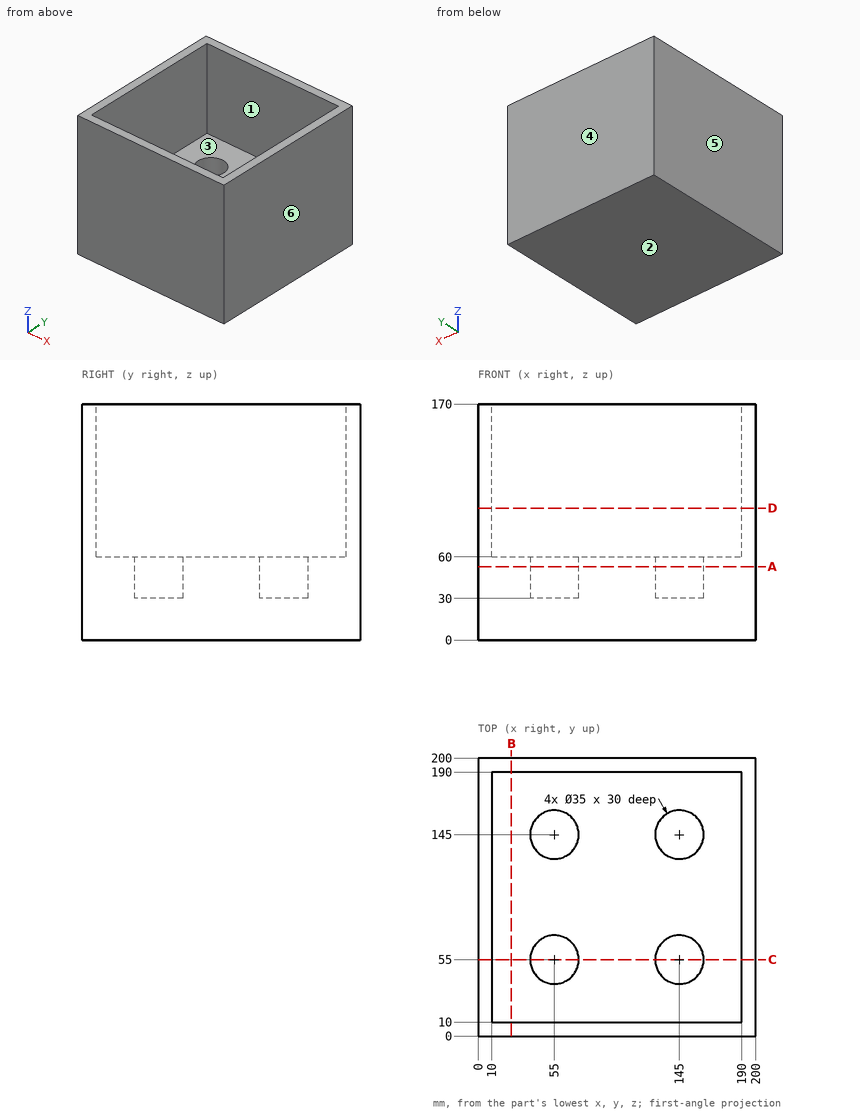
Print and shaded views of the part. All mm, measured from the part's lowest x, y and z. A direction names the side the tool comes from. Coordinates: 2 decimals unless noted, no trailing zeros. Loops run counter-clockwise (first coordinate to the right, second up) from the corner with the lowest first, then second, coordinate; pieces in that order, holes last. Notation, with made-up numbers: (67.5, -27) -> (81.5, -27) arc R33 cw to (81.5, 9) -> close; hole circle Ø6 at (23, 42). An arc over 180 degrees is marked (long way). Use a Markdown table: item, result. Add a question column.
Item 1: Band-saw the part on C-C on y = 55. Write the cut outline in (x, z), plus the area to 3 significant figures.
Item 2: Band-saw the part on B-B on x = 24. Write the cut outline in (y, z), plus the area to 3 significant figures.
Item 3: Probe probe 1 along Y at (x, z) = (145, 45); probe 2 along Y at (x, z) = (18, 112). List the from-to ranges inside material, lowest first.
Item 4: Band-saw the part on A-A on z = 53. Write the cut outline in (x, y).
Item 5: Band-saw the part on D-D on z = 95. Write the cut outline in (x, y), plus the area to 3 significant figures.
Item 6: Flat gauge pins, fed straight in: P1, Ø10.5, axis at x = 146, y = 51, coming from the +Z side; P2, Ø4, axis at x = 26, y = 57, coming from the +Z side. Where does each tip first touch, or does it go through?
Item 7: Pull direction X, two halves, no side cores. Call the marked faces 3, 4, 5 and 6: +X half, -X half, draft (parallel to the pull), parting line (faces both ways), or undercut.
Item 8: Which spindle directions (+Z, -Z, +X, -X, +Y, -Y) get a long thin tool onto all of the face, cutting with end or side? Do the marked faces 1 and 2. Say none if no direction does.
Geometry says:
| question | item | result |
|---|---|---|
| 1 | outline | (0, 0) -> (200, 0) -> (200, 170) -> (190, 170) -> (190, 60) -> (162.5, 60) -> (162.5, 30) -> (127.5, 30) -> (127.5, 60) -> (72.5, 60) -> (72.5, 30) -> (37.5, 30) -> (37.5, 60) -> (10, 60) -> (10, 170) -> (0, 170) -> close |
| 1 | area | 12,100 mm² |
| 2 | outline | (0, 0) -> (200, 0) -> (200, 170) -> (190, 170) -> (190, 60) -> (10, 60) -> (10, 170) -> (0, 170) -> close |
| 2 | area | 14,200 mm² |
| 3 | probe 1 | 0 to 37.5, 72.5 to 127.5, 162.5 to 200 |
| 3 | probe 2 | 0 to 10, 190 to 200 |
| 4 | outline | (0, 0) -> (200, 0) -> (200, 200) -> (0, 200) -> close; hole circle Ø35 at (55, 55); hole circle Ø35 at (55, 145); hole circle Ø35 at (145, 55); hole circle Ø35 at (145, 145) |
| 5 | outline | (0, 0) -> (200, 0) -> (200, 200) -> (0, 200) -> close; hole (10, 10) -> (190, 10) -> (190, 190) -> (10, 190) -> close |
| 5 | area | 7,600 mm² |
| 6 | P1 | z = 30 |
| 6 | P2 | z = 60 |
| 7 | face 3 | undercut |
| 7 | face 4 | draft |
| 7 | face 5 | -X half |
| 7 | face 6 | +X half |
| 8 | face 1 | +Z |
| 8 | face 2 | -Z, +X, -X, +Y, -Y |
